The figure shows three views and two pictorial views of one solid part (mm, origin at its lowest corner). Answer the questions. Coordinates: 2 decimals unless noted, no trailing zeros. Loops run counter-clockwise (first coordinate to the right, second up) from the corner with the lowest first, then second, coordinate; pieces in that order, holes last. Notation, with made-up numbers: M 6.25,45.5 L 23.25,45.5 A29 ccw 23.25,79.5 Z; hole C 21.5,-9 d4. An arc over 180 degrees is marked long. Return JSON: item names as keys, results as strings. Group by question number.
1. Straight lines are drawn through the part: L1, parallel to X at y = 1.15, z = 50; L2, parallel to Z at x = 66.5, y = 4.15 (3 decimals). For each, find the intervals that lie inside material, in ascending order. Write a range as from..to.
2. Section B-B (y = 2.9) is taken. Count the separate pieces of the cut face and the enclosed holes in it, then the cut area to 3 significant figures.
3. Section A-A (z = 50) is taken. Write down the section's boundary in (x, y), then the cut area to 4 significant figures.
4. Section C-C (x = 19) is taken. Write down the section's boundary in (y, z), then the cut area to 3 significant figures.
5. Given P1, Ø2.5, axis at x = 68, y = 2.5, coming from the -Z side; P2, Ø3, axis at y = 4, z = 35, coming from the +X side; P3, Ø2.5, axis at y = 3, z = 23, coming from the -X side; P4, Ø3.5, axis at x = 44, z = 50, coming from the -Y side, each flat-ended and moving along its own axis, determine where each tip first touches the part or whether it passes through.
6. Section D-D (x = 56) is taken. Write down the section's boundary in (y, z), then the cut area to 3 significant figures.
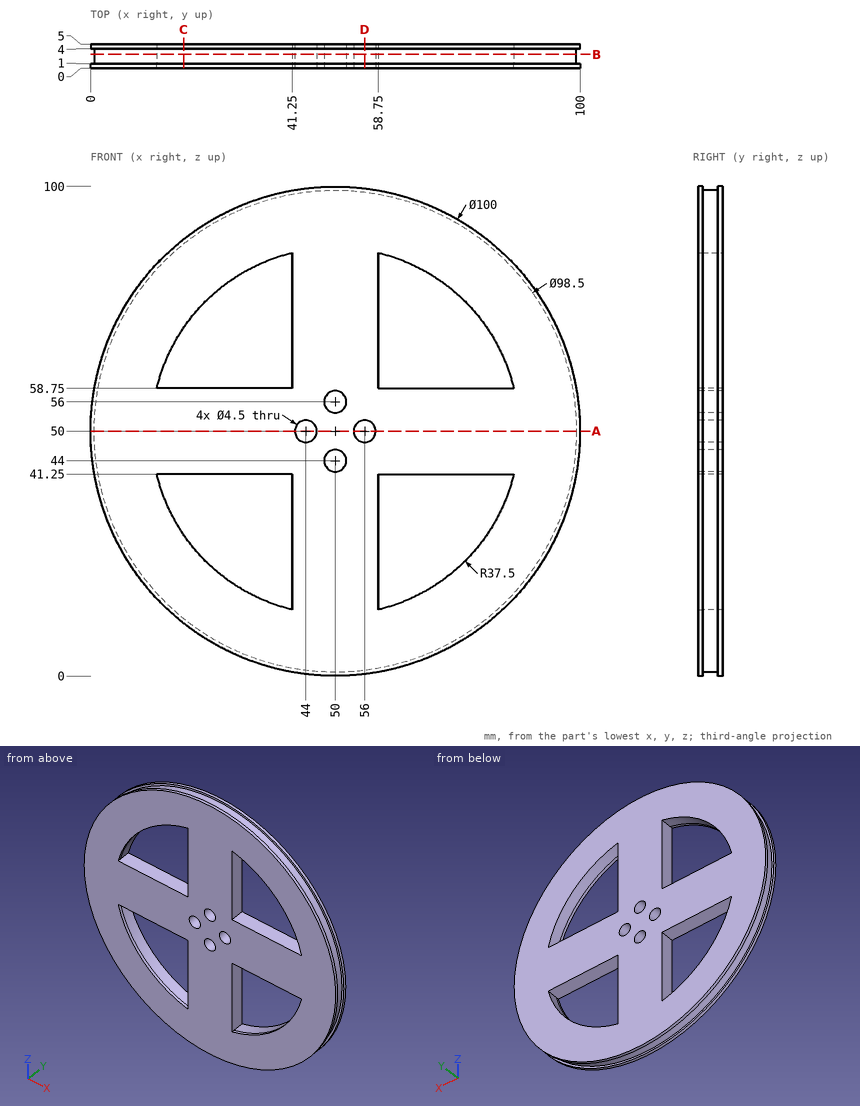
Worked out:
{
 "1": {"L1": "0.75..41.75, 46.25..53.75, 58.25..99.25", "L2": "2.801..16.325, 41.25..58.75, 83.675..97.199"},
 "2": {"separate pieces": "1", "enclosed holes": "8", "area": "5,430 mm^2"},
 "3": {"outline": "M 0,0 L 41.75,0 L 41.75,5 L 0,5 L 0,4 L 0.75,4 L 0.75,1 L 0,1 Z; M 46.25,0 L 53.75,0 L 53.75,5 L 46.25,5 Z; M 58.25,0 L 100,0 L 100,1 L 99.25,1 L 99.25,4 L 100,4 L 100,5 L 58.25,5 Z", "area": "450.5 mm^2"},
 "4": {"outline": "M 0,10.77 L 1,10.77 L 1,11.73 L 4,11.73 L 4,10.77 L 5,10.77 L 5,28.9 L 0,28.9 Z; M 0,41.25 L 5,41.25 L 5,58.75 L 0,58.75 Z; M 0,71.1 L 5,71.1 L 5,89.23 L 4,89.23 L 4,88.27 L 1,88.27 L 1,89.23 L 0,89.23 Z", "area": "263 mm^2"},
 "5": {"P1": "z = 3.69", "P2": "x = 98.14", "P3": "x = 7.44", "P4": "through"},
 "6": {"outline": "M 0,0.36 L 1,0.36 L 1,1.12 L 4,1.12 L 4,0.36 L 5,0.36 L 5,47.75 L 0,47.75 Z; M 0,52.25 L 5,52.25 L 5,99.64 L 4,99.64 L 4,98.88 L 1,98.88 L 1,99.64 L 0,99.64 Z", "area": "469 mm^2"}
}
